```python
from build123d import *

# Parameters (mm, degrees)
SKETCH002_R      = 1.25
EXTRUDE002_DEPTH = 10
SKETCH001_W      = 21
SKETCH001_H      = 2.85
EXTRUDE001_DEPTH = 12
EXTRUDE_DEPTH    = 10


with BuildPart() as extrude002:
    # Sketch002 (on Face5 of Cut) → Extrude002 (new body)
    with BuildSketch(Plane.XY.offset(10)):
        with Locations((32.341689, 32.041152)):
            Circle(SKETCH002_R)
        with Locations((38.850059, 22.11452)):
            Circle(SKETCH002_R)
    extrude(amount=-EXTRUDE002_DEPTH)


with BuildPart() as extrude001:
    # Sketch001 (on Face1 of Extrude) → Extrude001 (new body)
    with BuildSketch(Plane(origin=(28.885191, 0, 0), x_dir=(0, -1, 0), z_dir=(-1, 0, 0))):
        with Locations((-25.598607, 5)):
            Rectangle(SKETCH001_W, SKETCH001_H)
    extrude(amount=-EXTRUDE001_DEPTH)


with BuildPart() as cut001:
    # Sketch → Extrude (new body)
    with BuildSketch(Plane.XY):
        Polygon((30.354899, 31.776263), (40.592222, 15.770101), (40.592222, 45.770101), (31.175097, 72.086635), (28.885191, 72.086635), (28.885191, 57.086635), (30.354899, 51.776263), align=None)
    extrude(amount=EXTRUDE_DEPTH)

    # Cut: cut Extrude001
    add(extrude001.part, mode=Mode.SUBTRACT)

    # Cut001: cut Extrude002
    add(extrude002.part, mode=Mode.SUBTRACT)


solid = cut001.part
```
Here's how the part is built. I have some questions about the finished solid (model axes, mm). A direction names the side the tool comes from. Coordinates: 2 decimals unless noted, no trailing zeros. Order: outer loops, then holes, each group sorted by start corner. A loop starts at its lowest first (then second) coordinate and runs counter-clockwise, first axis right, second up. Notation, with made-up numbers: (73.25, 1) -> (106.25, 1) arc R8 ccw to (106.25, 10) -> close; hole circle Ø4 at (-35.5, 78.5). An arc over 180 degrees is marked (long way). Return JSON: item names as keys, results as strings.
1) On a 3-axis mill with a long thin cutter (end or side, diameter ignored), from which of +Z, -Z, +X, -X, +Y, -Y can I reach the whole of each face in a straight line? I mean faces 1 (the flat face through (30.355, 42, 5)), 2 (the flat face through (37, 28, 6.425)), 3 (the cylindrical face through (31.093, 32.096, 1.813)). Say none if no direction works.
Conclusion:
{"face 1": "+Z, -Z, -X, -Y", "face 2": "+X, -X, -Y", "face 3": "+Z, -Z"}
2) If we section it at A-A on y = 35: List the corners of the cut face in (x, z) for me (3 decimals).
Conclusion:
{"outline": "(30.355, 0) -> (40.592, 0) -> (40.592, 3.575) -> (30.355, 3.575) -> close; (30.355, 6.425) -> (40.592, 6.425) -> (40.592, 10) -> (30.355, 10) -> close"}
3) If we section it at B-B on z = 4.75: List the corners of the cut face in (x, y) for me, plus the area to 3 significant figures.
Conclusion:
{"outline": "(28.89, 57.09) -> (30.35, 51.78) -> (30.35, 36.1) -> (40.59, 36.1) -> (40.59, 45.77) -> (31.18, 72.09) -> (28.89, 72.09) -> close", "area": "270 mm²"}
4) Thinking about a two-plate mould opening in Z: for faces 4 (the flat face through (37, 28, 3.575)), 5 (the flat face through (35, 36.099, 5)), 6 (the flat face through (35, 44, 0)), 7 (the flat face through (29.6, 54.5, 4.9)), which applies, +Z half, -Z half, draft (parallel to the pull), parting line (faces both ways), or undercut?
Conclusion:
{"face 4": "undercut", "face 5": "undercut", "face 6": "-Z half", "face 7": "draft"}
5) If I drill on probe 1 along Z at (x, y) = (38.25, 23.5) (3 decimals); probe 2 along X at (y, z) = (43.5, 3.75); probe 3 along X at (y, z) = (49, 9.5), over which ranges is the centre line in solid material (lowest first)?
Conclusion:
{"probe 1": "z = 0 to 3.575, 6.425 to 10", "probe 2": "x = 30.35 to 40.59", "probe 3": "x = 30.35 to 39.44"}
6) I'm going to push flat-ended pins straight in: P1, Ø0.9, axis at x = 34, z = 5, coming from the -Y side; P2, Ø2, axis at y = 61.5, z = 8.5, coming from the +X side; P3, Ø2, axis at x = 32.34, y = 32.04, coming from the +Z side; P4, Ø1, axis at x = 37, z = 2.5, coming from the -Y side. Where does each tip first touch, or does it pass through?
Conclusion:
{"P1": "stops at y = 36.1", "P2": "stops at x = 35.32", "P3": "passes through", "P4": "stops at y = 20.6"}
7) If we section it at C-C on z = 9.5: List the corners of the cut face in (x, y) for me.
Conclusion:
{"outline": "(28.89, 57.09) -> (30.35, 51.78) -> (30.35, 31.78) -> (40.59, 15.77) -> (40.59, 45.77) -> (31.18, 72.09) -> (28.89, 72.09) -> close; hole circle Ø2.5 at (32.34, 32.04); hole circle Ø2.5 at (38.85, 22.11)"}
8) If we section it at D-D on y = 43: List the corners of the cut face in (x, z) for me, plus the area to 3 significant figures.
Conclusion:
{"outline": "(30.35, 0) -> (40.59, 0) -> (40.59, 10) -> (30.35, 10) -> close", "area": "102 mm²"}
